For this review, take the finished solid that the model builds, in its own axes (mm). A direction names the side the tool comes from. Coordinates: 2 decimals unless noted, no trailing zeros. Order: outer loops, then holes, each group sorted by start corner. A loop starts at its lowest first (then second) coordinate and runs counter-clockwise, first axis right, second up. Notation, with made-up numbers: (35.25, 46) -> (90.25, 46) arc R25 ccw to (90.25, 69) -> close; hole circle Ø3 at (50, 60). An arc over 180 degrees is marked (long way). Answer as a JSON object with one key per item and string values. Group by question number.
1) Wall thickness on L1, parallel to Y at x = 6.75, z = 72 (3 decimals); L2, parallel to Z at x = 0.75, y = -29.5; L3, parallel to Z at x = 2.75, y = -68 (3 decimals): over which ranges is each line inside the solid? List them lowest first.
2) Draft analysis for pull direction Y (two halves, no side actions). For faces 5 (the flat face through (10, -64, 61)), 6 (the cylindrical face through (4.93, -69.265, 50.027)), 7 (the cylindrical face through (1.972, -78.605, 57.657)), state which applies: +Y half, -Y half, draft (parallel to the pull), parting line (faces both ways), or undercut.
3) Add section C-C, the plane y = -78. Write out the cut boundary in (x, z), then the cut area to 3 significant figures.
4) Add section B-B, the plane y = -25.5. Write out the cut boundary in (x, z), then the cut area to 3 significant figures.
5) For pin 1 (2 mm diameter, centred on y = -68, z = 72, fed in from +X); pin 2 (1.2 mm diameter, centred on y = -88, z = 72, fed in from +X); pin 3 (1.2 mm diameter, centred on x = 2.5, z = 7.5, fed in from +Y); pin 4 (2 mm diameter, centred on y = -40, z = 70, fed in from -X), all flat-tipped, find the tip position at first contact; note any pin that passes through.
6) Add section A-A, the plane x = 8.5. Write out the cut boundary in (y, z) (3 decimals).
7) Machinability: for faces 1 (the cylindrical face through (3.254, -98.028, 63.5)), 2 (the cylindrical face through (4.289, -94.028, 72.196)), 3 (the flat face through (5, -84, 10)), 4 (the flat face through (2, -96, 8)), which of the approach directions +Z, -Z, +X, -X, +Y, -Y give a long, thin tool a straight path to every point of the face, cutting with its end or side? Answer none if there is none.
from build123d import *

# Parameters (mm, degrees)
PAD003_DEPTH    = 10
POCKET003_DEPTH = 4
SKETCH008_R     = 0.775
POCKET004_DEPTH = 10.001
FILLET_R        = 4
POCKET005_DEPTH = 8
PAD004_DEPTH    = 4


with BuildPart() as part:
    # Sketch006 → Pad003 (new body)
    with BuildSketch(Plane.YZ):
        with BuildLine():
            Line((-100, 80), (15, 80))
            Line((15, 80), (15, 64))
            Line((15, 64), (-35, 64))
            ThreePointArc((-35, 64), (-69.648232, 49.648232), (-84, 15))
            Line((-84, 15), (-84, 0))
            Line((-84, 0), (-100, 0))
            Line((-100, 0), (-100, 80))
        make_face()
    extrude(amount=PAD003_DEPTH)

    # Sketch007 (on Face8 of Pad003) → Pocket003 (cut)
    with BuildSketch(Plane(origin=(0, 0, 0), x_dir=(0, 1, 0), z_dir=(-1, 0, 0))):
        with BuildLine():
            Line((-88, 0), (-88, -15))
            ThreePointArc((-88, -15), (-72.476659, -52.476659), (-35, -68))
            Line((-35, -68), (-8, -68))
            ThreePointArc((-8, -68), (-5.171573, -66.828427), (-4, -64))
            Line((-4, -64), (4, -64))
            ThreePointArc((-8, -76), (0.485281, -72.485281), (4, -64))
            Line((-8, -76), (-35, -76))
            ThreePointArc((-96, -15), (-78.133514, -58.133514), (-35, -76))
            Line((-96, -15), (-96, 0))
            Line((-96, 0), (-88, 0))
        make_face()
    extrude(amount=-POCKET003_DEPTH, mode=Mode.SUBTRACT)

    # Sketch008 (on Face4 of Pocket003) → Pocket004 (cut, through all)
    with BuildSketch(Plane(origin=(0, 0, 0), x_dir=(0, 1, 0), z_dir=(-1, 0, 0))):
        with Locations((-88, -52)):
            Circle(SKETCH008_R)
        with Locations((-68, -72)):
            Circle(SKETCH008_R)
        with Locations((-88, -72)):
            Circle(SKETCH008_R)
        with Locations((7, -72)):
            Circle(SKETCH008_R)
    extrude(amount=-POCKET004_DEPTH, mode=Mode.SUBTRACT)

    # Fillet
    fillet_edges = [part.edges().sort_by_distance(p)[0] for p in [
        (5, 15, 64),
        (5, 15, 80),
        (5, -100, 80),
        (5, -100, 0),
        (5, -84, 0),
    ]]
    fillet(fillet_edges, radius=FILLET_R)

    # Sketch009 (on Face6 of Fillet) → Pocket005 (cut)
    with BuildSketch(Plane(origin=(0, -100, 0), x_dir=(0, 0, -1), z_dir=(0, -1, 0))):
        with BuildLine():
            ThreePointArc((-68, 6), (-74, 0), (-68, -6))
            Line((-68, -6), (-58, -6))
            ThreePointArc((-58, -6), (-52, 0), (-58, 6))
            Line((-68, 6), (-58, 6))
        make_face()
    extrude(amount=-POCKET005_DEPTH, mode=Mode.SUBTRACT)

    # Sketch010 (on Face14 of Pocket005) → Pad004 (join)
    with BuildSketch(Plane(origin=(0, -100, 0), x_dir=(0, 0, -1), z_dir=(0, -1, 0))):
        with BuildLine():
            ThreePointArc((-71, 3), (-73.12132, 2.12132), (-74, 0))
            ThreePointArc((-68, 6), (-72.242641, 4.242641), (-74, 0))
            Line((-58, 6), (-68, 6))
            ThreePointArc((-58, 6), (-60.44949, 5.477226), (-62.472136, 4))
            ThreePointArc((-64.708204, 3), (-63.483459, 3.261387), (-62.472136, 4))
            Line((-71, 3), (-64.708204, 3))
        make_face()
    extrude(amount=-PAD004_DEPTH)


solid = part.part
Output values:
{
 "1": {"L1": "y = -100 to -88.775, -87.225 to -68.775, -67.225 to 6.225, 7.775 to 15", "L2": "z = 64 to 68, 76 to 80", "L3": "z = 51.222 to 56.473, 66.303 to 71.225, 72.775 to 80"},
 "2": {"face 5": "draft", "face 6": "+Y half", "face 7": "undercut"},
 "3": {"outline": "(0, 38.49) -> (10, 38.49) -> (10, 80) -> (0, 80) -> (0, 58.27) -> (4, 58.27) -> (4, 45.98) -> (0, 45.98) -> close", "area": "366 mm²"},
 "4": {"outline": "(0, 64) -> (10, 64) -> (10, 80) -> (0, 80) -> (0, 76) -> (4, 76) -> (4, 68) -> (0, 68) -> close", "area": "128 mm²"},
 "5": {"pin 1": "stops at x = 10", "pin 2": "passes through", "pin 3": "stops at y = -84", "pin 4": "stops at x = 4"},
 "6": {"outline": "(-100, 4) arc R4 ccw to (-96, 0) -> (-88, 0) arc R4 ccw to (-84, 4) -> (-84, 15) arc R49 cw to (-35, 64) -> (11, 64) arc R4 ccw to (15, 68) -> (15, 76) arc R4 ccw to (11, 80) -> (-96, 80) arc R4 ccw to (-100, 76) -> close; hole circle Ø1.55 at (-88, 52); hole circle Ø1.55 at (-88, 72); hole circle Ø1.55 at (-68, 72); hole circle Ø1.55 at (7, 72)"},
 "7": {"face 1": "-X, -Y", "face 2": "-X", "face 3": "-Z, +X, -X, +Y", "face 4": "-Z, -X"}
}
